from build123d import *

# Parameters (mm, degrees)
F0_R     = 34.7
F1_DEPTH = 12.5
F2_R     = 12.7
F3_DEPTH = 25


with BuildPart() as f1:
    # F0 (on Top) → F1 (new body)
    with BuildSketch(Plane.XY):
        with BuildLine():
            ThreePointArc((18.962381, 107.541007), (18.732532, 115.603405), (21.706022, 123.100969))
            ThreePointArc((21.706022, 123.100969), (8.92339, 119.163541), (0, 109.2))
            ThreePointArc((0, 109.2), (-1.626378, 117.1), (0, 125))
            ThreePointArc((0, 125), (-11.904708, 118.902709), (-18.962381, 107.541007))
            ThreePointArc((-18.962381, 107.541007), (-21.935871, 115.03857), (-21.706022, 123.100969))
            ThreePointArc((-21.706022, 123.100969), (-32.371088, 115.029079), (-37.3486, 102.614434))
            ThreePointArc((-37.3486, 102.614434), (-41.578854, 109.481752), (-42.752518, 117.461578))
            ThreePointArc((-42.752518, 117.461578), (-51.853888, 107.660348), (-54.6, 94.569974))
            ThreePointArc((-54.6, 94.569974), (-59.958484, 100.598386), (-62.5, 108.253175))
            ThreePointArc((-62.5, 108.253175), (-69.761134, 97.020413), (-70.192407, 83.652053))
            ThreePointArc((-70.192407, 83.652053), (-76.516307, 88.658389), (-80.348451, 95.755555))
            ThreePointArc((-80.348451, 95.755555), (-85.548724, 83.432561), (-83.652053, 70.192407))
            ThreePointArc((-83.652053, 70.192407), (-90.74922, 74.024552), (-95.755555, 80.348451))
            ThreePointArc((-95.755555, 80.348451), (-98.736959, 67.309653), (-94.569974, 54.6))
            ThreePointArc((-94.569974, 54.6), (-102.224764, 57.141516), (-108.253175, 62.5))
            ThreePointArc((-108.253175, 62.5), (-108.925121, 49.141575), (-102.614434, 37.3486))
            ThreePointArc((-102.614434, 37.3486), (-110.59426, 38.522264), (-117.461578, 42.752518))
            ThreePointArc((-117.461578, 42.752518), (-115.803648, 29.480355), (-107.541007, 18.962381))
            ThreePointArc((-107.541007, 18.962381), (-115.603405, 18.732532), (-123.100969, 21.706022))
            ThreePointArc((-123.100969, 21.706022), (-119.163541, 8.92339), (-109.2, 0))
            ThreePointArc((-109.2, 0), (-117.1, -1.626378), (-125, 0))
            ThreePointArc((-125, 0), (-118.902709, -11.904708), (-107.541007, -18.962381))
            ThreePointArc((-107.541007, -18.962381), (-115.03857, -21.935871), (-123.100969, -21.706022))
            ThreePointArc((-123.100969, -21.706022), (-115.029079, -32.371088), (-102.614434, -37.3486))
            ThreePointArc((-102.614434, -37.3486), (-109.481752, -41.578854), (-117.461578, -42.752518))
            ThreePointArc((-117.461578, -42.752518), (-107.660348, -51.853888), (-94.569974, -54.6))
            ThreePointArc((-94.569974, -54.6), (-100.598386, -59.958484), (-108.253175, -62.5))
            ThreePointArc((-108.253175, -62.5), (-97.020413, -69.761134), (-83.652053, -70.192407))
            ThreePointArc((-83.652053, -70.192407), (-88.658389, -76.516307), (-95.755555, -80.348451))
            ThreePointArc((-95.755555, -80.348451), (-83.432561, -85.548724), (-70.192407, -83.652053))
            ThreePointArc((-70.192407, -83.652053), (-74.024552, -90.74922), (-80.348451, -95.755555))
            ThreePointArc((-80.348451, -95.755555), (-67.309653, -98.736959), (-54.6, -94.569974))
            ThreePointArc((-54.6, -94.569974), (-57.141516, -102.224764), (-62.5, -108.253175))
            ThreePointArc((-62.5, -108.253175), (-49.141575, -108.925121), (-37.3486, -102.614434))
            ThreePointArc((-37.3486, -102.614434), (-38.522264, -110.59426), (-42.752518, -117.461578))
            ThreePointArc((-42.752518, -117.461578), (-29.480355, -115.803648), (-18.962381, -107.541007))
            ThreePointArc((-18.962381, -107.541007), (-18.732532, -115.603405), (-21.706022, -123.100969))
            ThreePointArc((-21.706022, -123.100969), (-8.92339, -119.163541), (0, -109.2))
            ThreePointArc((0, -109.2), (1.626378, -117.1), (0, -125))
            ThreePointArc((0, -125), (11.904708, -118.902709), (18.962381, -107.541007))
            ThreePointArc((18.962381, -107.541007), (21.935871, -115.03857), (21.706022, -123.100969))
            ThreePointArc((21.706022, -123.100969), (32.371088, -115.029079), (37.3486, -102.614434))
            ThreePointArc((37.3486, -102.614434), (41.578854, -109.481752), (42.752518, -117.461578))
            ThreePointArc((42.752518, -117.461578), (51.853888, -107.660348), (54.6, -94.569974))
            ThreePointArc((54.6, -94.569974), (59.958484, -100.598386), (62.5, -108.253175))
            ThreePointArc((62.5, -108.253175), (69.761134, -97.020413), (70.192407, -83.652053))
            ThreePointArc((70.192407, -83.652053), (76.516307, -88.658389), (80.348451, -95.755555))
            ThreePointArc((80.348451, -95.755555), (85.548724, -83.432561), (83.652053, -70.192407))
            ThreePointArc((83.652053, -70.192407), (90.74922, -74.024552), (95.755555, -80.348451))
            ThreePointArc((95.755555, -80.348451), (98.736959, -67.309653), (94.569974, -54.6))
            ThreePointArc((94.569974, -54.6), (102.224764, -57.141516), (108.253175, -62.5))
            ThreePointArc((108.253175, -62.5), (108.925121, -49.141575), (102.614434, -37.3486))
            ThreePointArc((102.614434, -37.3486), (110.59426, -38.522264), (117.461578, -42.752518))
            ThreePointArc((117.461578, -42.752518), (115.803648, -29.480355), (107.541007, -18.962381))
            ThreePointArc((107.541007, -18.962381), (115.603405, -18.732532), (123.100969, -21.706022))
            ThreePointArc((123.100969, -21.706022), (119.163541, -8.92339), (109.2, 0))
            ThreePointArc((109.2, 0), (117.1, 1.626378), (125, 0))
            ThreePointArc((125, 0), (118.902709, 11.904708), (107.541007, 18.962381))
            ThreePointArc((107.541007, 18.962381), (115.03857, 21.935871), (123.100969, 21.706022))
            ThreePointArc((123.100969, 21.706022), (115.029079, 32.371088), (102.614434, 37.3486))
            ThreePointArc((102.614434, 37.3486), (109.481752, 41.578854), (117.461578, 42.752518))
            ThreePointArc((117.461578, 42.752518), (107.660348, 51.853888), (94.569974, 54.6))
            ThreePointArc((94.569974, 54.6), (100.598386, 59.958484), (108.253175, 62.5))
            ThreePointArc((108.253175, 62.5), (97.020413, 69.761134), (83.652053, 70.192407))
            ThreePointArc((83.652053, 70.192407), (88.658389, 76.516307), (95.755555, 80.348451))
            ThreePointArc((95.755555, 80.348451), (83.432561, 85.548724), (70.192407, 83.652053))
            ThreePointArc((70.192407, 83.652053), (74.024552, 90.74922), (80.348451, 95.755555))
            ThreePointArc((80.348451, 95.755555), (67.309653, 98.736959), (54.6, 94.569974))
            ThreePointArc((54.6, 94.569974), (57.141516, 102.224764), (62.5, 108.253175))
            ThreePointArc((62.5, 108.253175), (49.141575, 108.925121), (37.3486, 102.614434))
            ThreePointArc((37.3486, 102.614434), (38.522264, 110.59426), (42.752518, 117.461578))
            ThreePointArc((42.752518, 117.461578), (29.480355, 115.803648), (18.962381, 107.541007))
        make_face()
        Circle(F0_R, mode=Mode.SUBTRACT)
    extrude(amount=F1_DEPTH)

    # F2 (on face) → F3 (cut)
    with BuildSketch(Plane.XY.offset(12.5)):
        with Locations((-0.491815, 70)):
            Circle(F2_R)
        with Locations((-60.375871, -35.425925)):
            Circle(F2_R)
        with Locations((60.867686, -34.574075)):
            Circle(F2_R)
    extrude(amount=-F3_DEPTH, mode=Mode.SUBTRACT)


solid = f1.part
Geometry: final body of the model. Coordinates: model frame, mm. Give positions to 0.01 mm unless a question says otherwise; leave off trailing zeros. Write each loop counter-clockwise with the first axis right and the second up, starting at its lowest first coordinate (ties: lowest second). Pieces come first, ordered by that corner, then holes.
(1) Mould query, pull axis X, two halves, no side actions, for faces 1 (the flat face through (26, -26, 0)), 2 (the cylindrical face through (9.083, 119.265, 6.162)). Classes: released by +X, released by -X, zero draft, split by the parting line, or undercut.
(2) Ray query, line 1 (Y direction, x = -9, z = 1.75); line 2 (Y direction, x = -61, z = 10.5); line 3 (X direction, y = 74, z = 11.5). Return the intervals inside material, ascending.
(3) Cut plane A-A, the plane x = 91. Return loops of the section in (y, z).
(4) Cut plane B-B, the plane y = 9.5. Return loops of the section in (x, z).
(5) Cut plane C-C, the plane z = 9.5. Give the number of separate pieces and of enclosed holes in the cut face, then the cut area to 3 significant figures.
(6) First-contact query: P1, Ø3, axis at y = -39.5, z = 2, coming from the +X side; P2, Ø20.5, axis at x = -0.49, y = 70, coming from the -Z side; P3, Ø3, axis at x = -93.5, z = 4, coming from the -Y side; P4, Ø3, axis at y = -26, z = 2.5, coming from the +X side. Flat tips, straight axial feed; report the tip coordinate or a pass-through.
Values follow:
1. face 1: zero draft
1. face 2: undercut
2. line 1: y = -119.21 to -33.51, 33.51 to 60.57, 79.43 to 121.2
2. line 2: y = -108.7 to -107.02, -97.62 to -48.11, -22.74 to 102.67
2. line 3: x = -98.14 to -90.72, -84.97 to -12.55, 11.56 to 86.15
3. outline: (-74.24, 0) - (70.86, 0) - (70.86, 12.5) - (-74.24, 12.5) - close; (78.21, 0) - (83.32, 0) - (83.32, 12.5) - (78.21, 12.5) - close
4. outline: (-119.52, 0) - (-33.37, 0) - (-33.37, 12.5) - (-119.52, 12.5) - close; (33.37, 0) - (120.86, 0) - (120.86, 12.5) - (33.37, 12.5) - close
5. separate pieces: 1
5. enclosed holes: 4
5. area: 39,000 mm2
6. P1: stops at x = 117.73
6. P2: passes through
6. P3: stops at y = -82.81
6. P4: stops at x = 114.87
